from build123d import *

# Parameters (mm, degrees)
SKETCH1_R               = 2.5
BOSS_EXTRUDE1_DEPTH     = 20
CUT_EXTRUDE1_DEPTH      = 5
CUT_EXTRUDE1_DEPTH_BACK = 5
SKETCH2_W               = 23.75
SKETCH2_H               = 48.430343558
SKETCH3_W               = 40
SKETCH3_H               = 3
BOSS_EXTRUDE2_DEPTH     = 18.668764839
CUT_EXTRUDE2_DEPTH      = 61.919773624
SKETCH5_W               = 6.668765996
SKETCH5_H               = 26
CUT_EXTRUDE3_DEPTH      = 20
FILLET1_R               = 0.5
FILLET3_START           = -4
FILLET3_DEPTH           = 28


with BuildPart() as part:
    # Sketch1 → Boss-Extrude1 (new body)
    with BuildSketch(Plane(origin=(0, 0, 0), x_dir=(1, 0, 0), z_dir=(0, 1, 0))):
        with BuildLine():
            Line((-20, 9.33438242), (20, 9.33438242))
            Line((20, 9.33438242), (20, -9.33438242))
            Line((20, -9.33438242), (3.75, -9.33438242))
            Line((3.75, -9.33438242), (3.75, -21.027193281))
            ThreePointArc((3.75, -21.027193281), (5, -24.33438242), (3.75, -27.641571559))
            Line((3.75, -27.641571559), (3.75, -43.027193281))
            ThreePointArc((3.75, -43.027193281), (0, -51.33438242), (-3.75, -43.027193281))
            Line((-3.75, -43.027193281), (-3.75, -27.641571559))
            ThreePointArc((-3.75, -27.641571559), (-5, -24.33438242), (-3.75, -21.027193281))
            Line((-3.75, -21.027193281), (-3.75, -9.33438242))
            Line((-3.75, -9.33438242), (-20, -9.33438242))
            Line((-20, -9.33438242), (-20, 9.33438242))
        make_face()
        with Locations(Location((0, -24.33438242, 0), (0, 0, 270))):
            Circle(SKETCH1_R, mode=Mode.SUBTRACT)
        with Locations(Location((0, -46.33438242, 0), (0, 0, 270))):
            Circle(SKETCH1_R, mode=Mode.SUBTRACT)
    extrude(amount=BOSS_EXTRUDE1_DEPTH)

    # Sketch2 → Cut-Extrude1 (cut, two sides: drawn at the far end of the back side and taken through both)
    with BuildSketch(Plane(origin=(0, 10, 0), x_dir=(1, 0, 0), z_dir=(0, 1, 0)).offset(-CUT_EXTRUDE1_DEPTH_BACK)):
        with Locations((0, -33.549554199)):
            Rectangle(SKETCH2_W, SKETCH2_H)
    extrude(amount=CUT_EXTRUDE1_DEPTH + CUT_EXTRUDE1_DEPTH_BACK, mode=Mode.SUBTRACT)

    # Sketch3 → Boss-Extrude2 (add)
    with BuildSketch(Plane.XY.offset(9.33438242)):
        with Locations((0, 21.5)):
            Rectangle(SKETCH3_W, SKETCH3_H)
    boss_extrude2 = extrude(amount=-BOSS_EXTRUDE2_DEPTH)

    # Mirror1: Boss-Extrude2 across plane
    add(boss_extrude2.mirror(Plane.ZX.offset(10)))

    # Sketch4 → Cut-Extrude2 (cut, through all)
    with BuildSketch(Plane(origin=(0, 23, 0), x_dir=(1, 0, 0), z_dir=(0, 1, 0))):
        Polygon((-20.060606499, 2.66561758), (0, -7.53438242), (19.99607118, 2.66561758), (20, 9.33438242), (-20, 9.33438242), align=None)
    extrude(amount=-CUT_EXTRUDE2_DEPTH, mode=Mode.SUBTRACT)

    # Sketch5 → Cut-Extrude3 (cut)
    with BuildSketch(Plane(origin=(19.994493824, 0, 0.011779509), x_dir=(-0.0005891375272774049, 0, 0.999999826458472), z_dir=(-0.9999998264584721, 0, -0.0005891375272774049))):
        with Locations((-6.011780552, 10)):
            Rectangle(SKETCH5_W, SKETCH5_H)
    extrude(amount=-CUT_EXTRUDE3_DEPTH, mode=Mode.SUBTRACT)

    # Fillet1
    # the kernel refuses this fillet: 0.5 mm, written as the material it takes off along each edge
    with BuildSketch(Plane(origin=(-20, -5.037877222, -2.634801648), x_dir=(0, 0, 1), z_dir=(0, 1, 0))) as fillet1_piece_1:
        with BuildLine():
            CenterArc((FILLET1_R * 1.6303017777, FILLET1_R), FILLET1_R, 153.048520929, 116.951479071)
            Line((FILLET1_R * 0.738911111215, FILLET1_R * 1.4532357882), (0, 0))
            Line((0, 0), (FILLET1_R * 1.6303017777, 0))
        make_face()
    extrude(amount=30.075754444, mode=Mode.SUBTRACT)
    with BuildSketch(Plane(origin=(20, 23.156386842, -2.665615266), x_dir=(0, 0, 1), z_dir=(0, -1, 0))) as fillet1_piece_2:
        with BuildLine():
            CenterArc((0.062554737, 0.5), FILLET1_R, 262.81265488, 7.18734512)
            Line((-2.315e-06, 0.00392882), (0, 0))
            Line((0, 0), (0.062554737, 0))
        make_face()
    extrude(amount=26.312773684, mode=Mode.SUBTRACT)

    # Fillet3: read off the stored shape, not the designer's step
    # Fillet3 outline → Fillet3 (cut)
    with BuildSketch(Plane(origin=(0, 0, 0), x_dir=(1, 0, 0), z_dir=(0, 1, 0)).offset(FILLET3_START)):
        with BuildLine():
            ThreePointArc((19.272801541, 2.296677589), (19.761152035, 2.277657587), (20, 1.851277926))
            Line((20, 1.851277926), (20, 2.603060529))
            ThreePointArc((20, 2.603060529), (19.999016828, 2.63440068), (19.99607118, 2.66561758))
            Line((19.99607118, 2.66561758), (19.272801541, 2.296677589))
        make_face()
    extrude(amount=FILLET3_DEPTH, mode=Mode.SUBTRACT)


solid = part.part
Could you check a few things on this model? Use its own coordinates, in mm. A direction names the side the tool comes from. Give positions to 0.01 mm unless a question says otherwise; leave off trailing zeros. Order: outer loops, then holes, each group sorted by start corner. A loop starts at its lowest first (then second) coordinate and runs counter-clockwise, first axis right, second up. Notation, with made-up numbers: (5, 37) - (44, 37) arc R10 ccw to (44, 41) - close; hole circle Ø5 at (88.5, 64.25). An arc over 180 degrees is marked (long way). One line per item, written item: value. Start each with the question number.
1. For P1, Ø10, axis at y = 5, z = 12, coming from the -X side; P2, Ø6, axis at x = 5.5, z = 17.5, coming from the +Y side; P3, Ø1.5, axis at y = 17, z = 15.5, coming from the -X side; P4, Ø5, axis at x = 1.5, z = 34.5, coming from the -Y side, each with a flat end and sliding along its axis, tell me the tip position at first contact or that it passes through.
2. Imagine slicing it at A-A on z = 18. List the corners of the cut face in (x, y) for me.
3. Thinking about a two-plate mould opening in X: for faces 5 (the face through (0.75, 17.46, 26.72)), 6 (the face through (3.75, 2, 35)), 7 (the face through (0, 5, 30)), which applies, +X half, -X half, draft (parallel to the pull), parting line (faces both ways), or undercut?
4. Imagine slicing it at D-D on y = 12.25. List the corners of the cut face in (x, z) for me, plus the area to 3 significant figures.
5. Imagine slicing it at B-B on y = 2.75. List the corners of the cut face in (x, z) for me.
6. Imagine slicing it at C-C on z = 25. List the corners of the cut face in (x, y) for me, plus the area to 3 significant figures.
7. For faces 1 (the face through (0, 0, 30)), 2 (the face through (9.5, 10.18, 2.69)), 3 (the face through (-3.75, 17, 35)), 4 (the face through (0, 20, 30)), which set-ups out of +Z, -Z, +X, -X, +Y, -Y let a thin tool reach every point of the face, with its end or its side?
8. If I drill on probe 1 along Z at (x, y) = (0, 18.3); probe 2 along Y at (x, z) = (0, 38.5); probe 3 along X at (y, z) = (19.5, 48.5), over which ranges is the centre line in solid material (lowest first)?
Values:
1. P1: x = -20
1. P2: y = 20
1. P3: x = -3.75
1. P4: y = 0
2. outline: (-3.75, 0) - (3.75, 0) - (3.75, 5) - (-3.75, 5) - close; (-3.75, 15) - (3.75, 15) - (3.75, 20) - (-3.75, 20) - close
3. face 5: undercut
3. face 6: +X half
3. face 7: draft
4. outline: (-20, -1.82) arc R0.5 ccw to (-19.27, -2.27) - (0, 7.53) - (19.27, -2.3) arc R0.5 ccw to (20, -1.85) - (20, 9.33) - (-20, 9.33) - close
4. area: 275 mm²
5. outline: (-20, -1.82) arc R0.5 ccw to (-19.27, -2.27) - (0, 7.53) - (19.27, -2.3) arc R0.5 ccw to (20, -1.85) - (20, 9.33) - (3.75, 9.33) - (3.75, 21.03) arc R5 ccw to (3.75, 27.64) - (3.75, 43.03) arc R5 ccw (long way) to (-3.75, 43.03) - (-3.75, 27.64) arc R5 ccw to (-3.75, 21.03) - (-3.75, 9.33) - (-20, 9.33) - close; hole circle Ø5 at (0, 24.33); hole circle Ø5 at (0, 46.33)
6. outline: (-4.96, 0) - (-2.41, 0) - (-2.41, 5) - (-4.96, 5) - close; (-4.96, 15) - (-2.41, 15) - (-2.41, 20) - (-4.96, 20) - close; (2.41, 0) - (4.96, 0) - (4.96, 5) - (2.41, 5) - close; (2.41, 15) - (4.96, 15) - (4.96, 20) - (2.41, 20) - close
6. area: 50.9 mm²
7. face 1: +Z, +X, -X, -Y
7. face 2: -Z, +Y, -Y
7. face 3: -X, +Y, -Y
7. face 4: +Z, +X, -X, +Y
8. probe 1: 7.53 to 21.83, 26.83 to 43.83, 48.83 to 51.33
8. probe 2: 0 to 5, 15 to 20
8. probe 3: -4.51 to -1.25, 1.25 to 4.51
